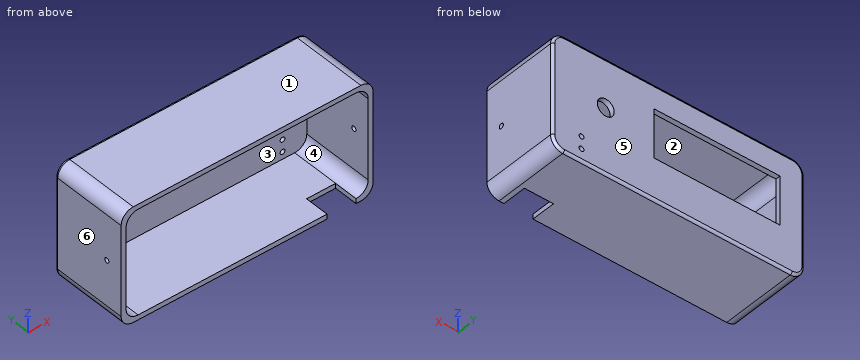
from build123d import *

# Parameters (mm, degrees)
SKETCH_1_R               = 3.5
SKETCH_1_R_2             = 1
SKETCH_1_W               = 52
SKETCH_1_H               = 20
EXTRUDE_1_DEPTH          = 2
EXTRUDE_2_DEPTH          = 32
FILLET_2_R               = 1
SKETCH_2_R               = 1
CUT_EXTRUDE_1_DEPTH      = 1
CUT_EXTRUDE_1_DEPTH_BACK = 105
SKETCH_3_W               = 12
SKETCH_3_H               = 10
CUT_EXTRUDE_2_DEPTH      = 10


with BuildPart() as part:
    # Эскиз1 → Бобышка-Вытянуть1 (new body)
    with BuildSketch(Plane(origin=(0, 0, 0), x_dir=(1, 0, 0), z_dir=(0, 1, 0))):
        with BuildLine():
            Line((-29, 25), (61, 25))
            ThreePointArc((61, 25), (64.535533906, 23.535533906), (66, 20))
            Line((66, 20), (66, -13))
            ThreePointArc((66, -13), (64.535533906, -16.535533906), (61, -18))
            Line((61, -18), (-29, -18))
            ThreePointArc((-29, -18), (-32.535533906, -16.535533906), (-34, -13))
            Line((-34, -13), (-34, 20))
            ThreePointArc((-34, 20), (-32.535533906, 23.535533906), (-29, 25))
        make_face()
        with Locations((46, 0)):
            Circle(SKETCH_1_R, mode=Mode.SUBTRACT)
        with Locations((56, 22)):
            Circle(SKETCH_1_R_2, mode=Mode.SUBTRACT)
        with Locations((56, 17)):
            Circle(SKETCH_1_R_2, mode=Mode.SUBTRACT)
        Rectangle(SKETCH_1_W, SKETCH_1_H, mode=Mode.SUBTRACT)
    extrude(amount=-EXTRUDE_1_DEPTH)

    # Эскиз1<3> → Бобышка-Вытянуть2 (add)
    with BuildSketch(Plane(origin=(0, 0, 0), x_dir=(1, 0, 0), z_dir=(0, 1, 0))):
        with BuildLine():
            Line((-31, 27), (63, 27))
            ThreePointArc((63, 27), (66.535533906, 25.535533906), (68, 22))
            Line((68, 22), (68, -15))
            ThreePointArc((68, -15), (66.535533906, -18.535533906), (63, -20))
            Line((63, -20), (-31, -20))
            ThreePointArc((-31, -20), (-34.535533906, -18.535533906), (-36, -15))
            Line((-36, -15), (-36, 22))
            ThreePointArc((-36, 22), (-34.535533906, 25.535533906), (-31, 27))
        make_face()
        with BuildLine():
            Line((-29, 25), (61, 25))
            ThreePointArc((61, 25), (64.535533906, 23.535533906), (66, 20))
            Line((66, 20), (66, -13))
            ThreePointArc((66, -13), (64.535533906, -16.535533906), (61, -18))
            Line((61, -18), (-29, -18))
            ThreePointArc((-29, -18), (-32.535533906, -16.535533906), (-34, -13))
            Line((-34, -13), (-34, 20))
            ThreePointArc((-34, 20), (-32.535533906, 23.535533906), (-29, 25))
        make_face(mode=Mode.SUBTRACT)
    extrude(amount=-EXTRUDE_2_DEPTH)

    # Скругление2
    fillet_2_edges = [part.edges().sort_by_distance(p)[0] for p in [
        (-34.535533906, 0, -25.535533906),
        (16, 0, -27),
        (68, 0, -3.5),
        (66.535533906, 0, 18.535533906),
        (-36, 0, -3.5),
        (-34.535533906, 0, 18.535533906),
        (16, 0, 20),
        (66.535533906, 0, -25.535533906),
    ]]
    fillet(fillet_2_edges, radius=FILLET_2_R)

    # Эскиз2 → Вырез-Вытянуть1 (cut, two sides)
    with BuildSketch(Plane(origin=(68, 0, 0), x_dir=(0, 0, -1), z_dir=(1, 0, 0))) as cut_extrude_1_sk:
        with Locations((3.5, -25)):
            Circle(SKETCH_2_R)
    extrude(amount=CUT_EXTRUDE_1_DEPTH, mode=Mode.SUBTRACT)
    extrude(cut_extrude_1_sk.sketch, amount=-CUT_EXTRUDE_1_DEPTH_BACK, mode=Mode.SUBTRACT)

    # Эскиз3 → Вырез-Вытянуть2 (cut)
    with BuildSketch(Plane.XY.offset(-25)):
        with Locations((55, -27)):
            Rectangle(SKETCH_3_W, SKETCH_3_H)
    extrude(amount=-CUT_EXTRUDE_2_DEPTH, mode=Mode.SUBTRACT)


solid = part.part
Could you check a few things on this model? Use its own coordinates, in mm. Face numbers are marked on the shaded views. A direction names the side the tool comes from. Give positions to 0.01 mm unless a question says otherwise; leave off trailing zeros. Order: outer loops, then holes, each group sorted by start corner. A loop starts at its lowest first (then second) coordinate and runs counter-clockwise, first axis right, second up.
1. We'd pull the mould along X, two halves only. Please class the marked faces 3, 4, 5 and 6: pulls with the +X half, pulls with the -X half, needs draft (parallel to the pull), parting line crosses it, or undercut.
2. Suppose I cut it at C-C (y = -25). List the corners of the cut face in (x, z) for me.
3. Suppose I cut it at D-D (x = 28). List the corners of the cut face in (y, z) for me.
4. Suppose I cut it at B-B (z = -17). List the corners of the cut face in (x, y) for me.
5. For the marked faces 1 and 2, which set-ups out of +Z, -Z, +X, -X, +Y, -Y let a thin tool reach every point of the face, with its end or its side?
6. Suppose I cut it at A-A (x = 46). List the corners of the cut face in (y, z) for me.
7. Will these pins go through, and if not, where does the flat tip stop? P1, Ø2, axis at x = 54, z = -26.5, coming from the -Y side; P2, Ø2.5, axis at x = 56, z = -17, coming from the +Y side; P3, Ø0.6, axis at y = -0.5, z = -4, coming from the +X side; P4, Ø2, axis at y = -24.5, z = -26, coming from the +X side.
8. I need wall thicknesses on L1, parallel to Z at x = 56, y = -1.15; L2, parallel to X at y = -15.5, z = -4; L3, parallel to Y at x = 66.85, z = -3.5. Which ranges of each line are inside material? Lowest first, please.
Solved:
1. face 3: undercut
1. face 4: undercut
1. face 5: needs draft
1. face 6: pulls with the -X half
2. outline: (-36, -22) arc R5 ccw to (-31, -27) - (49, -27) - (49, -25) - (-29, -25) arc R5 cw to (-34, -20) - (-34, -4.5) - (-36, -4.5) - close; (-36, -2.5) - (-34, -2.5) - (-34, 13) arc R5 cw to (-29, 18) - (61, 18) arc R5 cw to (66, 13) - (66, -2.5) - (68, -2.5) - (68, 15) arc R5 ccw to (63, 20) - (-31, 20) arc R5 ccw to (-36, 15) - close; (61, -27) - (63, -27) arc R5 ccw to (68, -22) - (68, -4.5) - (66, -4.5) - (66, -20) arc R5 cw to (61, -25) - close
3. outline: (-32, -27) - (-1, -27) arc R1 ccw to (0, -26) - (0, 19) arc R1 ccw to (-1, 20) - (-32, 20) - (-32, 18) - (-2, 18) - (-2, -25) - (-32, -25) - close
4. outline: (-36, -32) - (-34, -32) - (-34, -2) - (55, -2) - (55, 0) - (-35, 0) arc R1 ccw to (-36, -1) - close; (57, -2) - (66, -2) - (66, -32) - (68, -32) - (68, -1) arc R1 ccw to (67, 0) - (57, 0) - close
5. face 1: +Z, +X, -X, +Y, -Y
5. face 2: -Y
6. outline: (-32, -27) - (-1, -27) arc R1 ccw to (0, -26) - (0, -3.5) - (-2, -3.5) - (-2, -25) - (-32, -25) - close; (-32, 18) - (-2, 18) - (-2, 3.5) - (0, 3.5) - (0, 19) arc R1 ccw to (-1, 20) - (-32, 20) - close
7. P1: stops at y = -22
7. P2: stops at y = 0
7. P3: stops at x = 67.98
7. P4: stops at x = 67
8. L1: z = -27 to -23, -21 to -18, -16 to 20
8. L2: x = -36 to -34, 66 to 68
8. L3: y = -32 to -26, -24 to 0
